Read the model definition and answer for the solid it produces. Units are mm, in the model's axes. A direction names the side the tool comes from. Coordinates: 2 decimals unless noted, no trailing zeros. Order: outer loops, then holes, each group sorted by start corner. A loop starts at its lowest first (then second) coordinate and runs counter-clockwise, first axis right, second up. Notation, with made-up numbers: (53, 80) - (71, 80) arc R33 ccw to (71, 108) - close; hole circle Ø11 at (25, 27.5). An arc over 180 degrees is marked (long way). Write item = value, one per line.
from build123d import *

# Parameters (mm, degrees)
F0_W            = 42.3
F0_H            = 42.3
F1_DEPTH        = 34
F2_R            = 11
F3_DEPTH        = 2
F4_R            = 2.5
F5_DEPTH        = 24
F6_R            = 2.25
F7_DEPTH        = 5
F7_COPIES_COUNT = 4
F8_SIZE         = 5


# Not quite as in the source:
# - a pattern or mirror of a feature is missing from the dataset's text; its kind, count and spacing are read off the source's solid


with BuildPart() as f1:
    # F0 (on Top) → F1 (new body)
    with BuildSketch(Plane.XY):
        Rectangle(F0_W, F0_H)
    extrude(amount=F1_DEPTH)

    # F2 (on face) → F3 (join)
    with BuildSketch(Plane.XY.offset(34)):
        Circle(F2_R)
    extrude(amount=F3_DEPTH)

    # F4 (on face) → F5 (join)
    with BuildSketch(Plane.XY.offset(36)):
        Circle(F4_R)
    extrude(amount=F5_DEPTH)

    # F6 (on face) → F7 (cut)
    with BuildSketch(Plane.XY.offset(34)):
        with Locations((-15.5, 15.5)):
            Circle(F6_R)
    f7 = extrude(amount=-F7_DEPTH, mode=Mode.SUBTRACT)

    # F7_copies: F7 ×4 about axis
    f7_copies_axis = Axis((0, 0, 0), (0, 0, 1))
    for i in range(1, F7_COPIES_COUNT):
        add(f7.rotate(f7_copies_axis, i * 360 / F7_COPIES_COUNT), mode=Mode.SUBTRACT)

    # F8
    f8_edges = [f1.edges().sort_by_distance(p)[0] for p in [
        (-21.15, -21.15, 17),
        (-21.15, 21.15, 17),
        (21.15, 21.15, 17),
        (21.15, -21.15, 17),
    ]]
    chamfer(f8_edges, length=F8_SIZE)


solid = f1.part
1) Flat-ended cylindrical pins translate along their axes: pin 1 Ø3.5 at (x, y) = (15.5, -15.5) entering from +Z; pin 2 Ø5 at (x, z) = (0.5, 41.5) entering from -Y; pin 3 Ø5 at (x, y) = (15.5, -16) entering from +Z. Find the tip coordinate at first contact, or state that the pin passes through.
Returned:
pin_1 = 29
pin_2 = -2.5
pin_3 = 34
2) The part is cut by section C-C (z = 28). Determine the outline of the cut face in (x, y).
Returned:
outline = (-21.15, -16.15) - (-16.15, -21.15) - (16.15, -21.15) - (21.15, -16.15) - (21.15, 16.15) - (16.15, 21.15) - (-16.15, 21.15) - (-21.15, 16.15) - close
3) Straight lines are drawn through the part: line 1 along X through (y, z) = (-15.5, 30.55); line 2 along Z through (x, y) = (15, -15.5). For each, find the intervals that lie inside material, in ascending order. Write a range as from..to.
Returned:
line_1 = -21.15..-17.75, -13.25..13.25, 17.75..21.15
line_2 = 0..29
4) Determine the mould class of faces 1 (the face through (13.504, 14.462, 31.535)), 2 (the face through (-18.6, -18.7, 16.8)), 3 (the face through (21.15, 0, 17)) for opening direction Y: pulls with the +Y half, pulls with the -Y half, needs draft (parallel to the pull), parting line crosses it, or undercut.
Returned:
face_1 = undercut
face_2 = pulls with the -Y half
face_3 = needs draft
5) The part is cut by section A-A (x = 0). Determine the outline of the cut face in (y, z), and give its area (3 significant figures).
Returned:
outline = (-21.15, 0) - (21.15, 0) - (21.15, 34) - (11, 34) - (11, 36) - (2.5, 36) - (2.5, 60) - (-2.5, 60) - (-2.5, 36) - (-11, 36) - (-11, 34) - (-21.15, 34) - close
area = 1,600 mm^2
6) For faces 4 (the face through (16, -16, 29)), 5 (the face through (-18.6, 18.7, 16.8)), determine the directions among +Z, -Z, +X, -X, +Y, -Y from which every point of the face is accessible in a straight line to the end or side of a thin tool.
Returned:
face_4 = +Z
face_5 = +Z, -Z, -X, +Y
7) The part is cut by section D-D (y = -7). Determine the outline of the cut face in (x, z).
Returned:
outline = (-21.15, 0) - (21.15, 0) - (21.15, 34) - (8.49, 34) - (8.49, 36) - (-8.49, 36) - (-8.49, 34) - (-21.15, 34) - close
